```python
from build123d import *

# Parameters (mm, degrees)
SKETCH_1_W          = 25
SKETCH_1_H          = 10
SKETCH_1_R          = 2.25
EXTRUDE_1_DEPTH     = 21.5
FILLET_1_R          = 2
SKETCH_2_W          = 8
SKETCH_2_H          = 13.5
CUT_EXTRUDE_1_DEPTH = 35.456494308
FILLET_2_R          = 1.5


with BuildPart() as part:
    # 草图1 → 凸台-拉伸1 (new body)
    with BuildSketch(Plane.XY):
        with Locations((12.5, 5)):
            Rectangle(SKETCH_1_W, SKETCH_1_H)
        with Locations((5, 5)):
            Circle(SKETCH_1_R, mode=Mode.SUBTRACT)
        with Locations((20, 5)):
            Circle(SKETCH_1_R, mode=Mode.SUBTRACT)
    extrude(amount=EXTRUDE_1_DEPTH)

    # 圆角1
    fillet_1_edges = [part.edges().sort_by_distance(p)[0] for p in [
        (0, 10, 10.75),
        (25, 10, 10.75),
        (25, 0, 10.75),
        (0, 0, 10.75),
    ]]
    fillet(fillet_1_edges, radius=FILLET_1_R)

    # 草图2 → 切除-拉伸1 (cut, through all)
    with BuildSketch(Plane(origin=(0, 10, 0), x_dir=(1, 0, 0), z_dir=(0, 1, 0))):
        with Locations((12.5, -10.75)):
            Rectangle(SKETCH_2_W, SKETCH_2_H)
    extrude(amount=-CUT_EXTRUDE_1_DEPTH, mode=Mode.SUBTRACT)

    # 圆角2
    fillet_2_edges = [part.edges().sort_by_distance(p)[0] for p in [
        (8.5, 0, 10.75),
        (8.5, 5, 17.5),
        (12.5, 0, 4),
        (8.5, 5, 4),
        (16.5, 0, 10.75),
        (16.5, 5, 4),
        (12.5, 0, 17.5),
        (16.5, 5, 17.5),
        (8.5, 10, 10.75),
        (12.5, 10, 17.5),
        (16.5, 10, 10.75),
        (12.5, 10, 4),
    ]]
    fillet(fillet_2_edges, radius=FILLET_2_R)


solid = part.part
```
Verification items for the finished model (mm, model axes). A direction names the side the tool comes from. Round coordinates to 2 decimals unless told otherwise and drop trailing zeros. Loops run counter-clockwise (first coordinate to the right, second up) from the corner with the lowest first, then second, coordinate; pieces in that order, holes last. Notation, with made-up numbers: (2.25, 45.25) -> (11.25, 45.25) arc R22 cw to (11.25, 65.25) -> close; hole circle Ø4 at (-33, 57). An arc over 180 degrees is marked (long way). Answer as a JSON object with one key per item and string values.
Q1. Section check C-C (x = 20). Record the boundary of the cut face in (y, z), then the cut area to 3 significant figures.
Data:
{"outline": "(0, 0) -> (2.75, 0) -> (2.75, 21.5) -> (0, 21.5) -> close; (7.25, 0) -> (10, 0) -> (10, 21.5) -> (7.25, 21.5) -> close", "area": "118 mm2"}
Q2. Scan lines: line 1 (Y direction, x = 20, z = 5); line 2 (X direction, y = 2.5, z = 9.75); line 3 (X direction, y = 4.5, z = 9). Record each from-to range of solid material in increasing order. Write a range as from..to.
Data:
{"line 1": "y = 0..2.75, 7.25..10", "line 2": "x = 0..8.5, 16.5..25", "line 3": "x = 0..2.81, 7.19..8.5, 16.5..17.81, 22.19..25"}
Q3. Section check D-D (x = 14.5). Record the boundary of the cut face in (y, z).
Data:
{"outline": "(0, 0) -> (10, 0) -> (10, 2.5) arc R1.5 ccw to (8.5, 4) -> (1.5, 4) arc R1.5 ccw to (0, 2.5) -> close; (0, 19) arc R1.5 ccw to (1.5, 17.5) -> (8.5, 17.5) arc R1.5 ccw to (10, 19) -> (10, 21.5) -> (0, 21.5) -> close"}
Q4. Section check B-B (z = 7). Record the boundary of the cut face in (x, y), then the cut area to 3 significant figures.
Data:
{"outline": "(0, 2) arc R2 ccw to (2, 0) -> (7, 0) arc R1.5 ccw to (8.5, 1.5) -> (8.5, 8.5) arc R1.5 ccw to (7, 10) -> (2, 10) arc R2 ccw to (0, 8) -> close; (16.5, 1.5) arc R1.5 ccw to (18, 0) -> (23, 0) arc R2 ccw to (25, 2) -> (25, 8) arc R2 ccw to (23, 10) -> (18, 10) arc R1.5 ccw to (16.5, 8.5) -> close; hole circle Ø4.5 at (5, 5); hole circle Ø4.5 at (20, 5)", "area": "133 mm2"}
Q5. Section check A-A (y = 5). Record the boundary of the cut face in (x, z), then the cut area to 3 significant figures.
Data:
{"outline": "(0, 0) -> (2.75, 0) -> (2.75, 21.5) -> (0, 21.5) -> close; (7.25, 0) -> (17.75, 0) -> (17.75, 21.5) -> (7.25, 21.5) -> close; (22.25, 0) -> (25, 0) -> (25, 21.5) -> (22.25, 21.5) -> close; hole (8.5, 5.5) arc R1.5 ccw to (10, 4) -> (15, 4) arc R1.5 ccw to (16.5, 5.5) -> (16.5, 16) arc R1.5 ccw to (15, 17.5) -> (10, 17.5) arc R1.5 ccw to (8.5, 16) -> close", "area": "238 mm2"}
Q6. Draft check along X on faces 1 (the cylindrical face through (8.05, 0.43, 10.68)), 2 (the flat face through (25, 5, 11)), 3 (the cylindrical face through (12.54, 9.57, 17.95)), 4 (the cylindrical face through (0.57, 9.4, 10.9)). Enter one of: pulls with the +X half, pulls with the -X half, needs draft (parallel to the pull), parting line crosses it, or undercut.
Data:
{"face 1": "undercut", "face 2": "pulls with the +X half", "face 3": "undercut", "face 4": "pulls with the -X half"}
Q7. Access from +Z, -Z, +X, -X, +Y, -Y to the whole of each face (thin tool, end or side, straight path). Record for faces 5 (the cylindrical face through (22.146, 5.676, 10.599)), 6 (the cylindrical face through (16.95, 9.57, 10.68)), 7 (the cylindrical face through (12.54, 0.43, 17.95)), 8 (the flat face through (5, 0, 11)), 9 (the cylindrical face through (8.95, 4.95, 4.43)).
Data:
{"face 5": "+Z, -Z", "face 6": "+Y", "face 7": "-Y", "face 8": "+Z, -Z, +X, -X, -Y", "face 9": "+Y, -Y"}
